Could you check a few things on this model? Use its own coordinates, in mm. A direction names the side the tool comes from. Give positions to 0.01 mm unless a question says otherwise; leave off trailing zeros. Order: outer loops, then holes, each group sorted by start corner. A loop starts at its lowest first (then second) coordinate and runs counter-clockwise, first axis right, second up. Notation, with made-up numbers: (22.5, -32) -> (59.5, -32) arc R17 cw to (59.5, -21) -> close; hole circle Ø6 at (52, 22). An arc over 180 degrees is marked (long way). Write each question's results on one line, items separated by ' | '.
```python
from build123d import *

# Parameters (mm, degrees)
F3_DEPTH      = 40.001
F3_DEPTH_BACK = 40.001
F4_R          = 20
F5_DEPTH      = 40.001
F5_DEPTH_BACK = 40.001


with BuildPart() as f1:
    # F0 (on Front) → F1 (revolve)
    with BuildSketch(Plane.XZ):
        with BuildLine():
            ThreePointArc((0, 40), (-40, 0), (0, -40))
            Line((0, -40), (0, 40))
        make_face()
    revolve(axis=Axis((0, 0, 0), (0, 0, 1)))

    # F2 (on Front) → F3 (cut, two sides)
    with BuildSketch(Plane.XZ) as f3_sk:
        Polygon((12.5, -25.9565174572), (28.0872450465, -6.4107303955), (22.5242216976, 17.9624674091), (0, 28.809560887), (-22.5242216976, 17.9624674091), (-28.0872450465, -6.4107303955), (-12.5, -25.9565174572), align=None)
    extrude(amount=-F3_DEPTH, mode=Mode.SUBTRACT)
    extrude(f3_sk.sketch, amount=F3_DEPTH_BACK, mode=Mode.SUBTRACT)

    # F4 (on Right) → F5 (cut, two sides)
    with BuildSketch(Plane.YZ) as f5_sk:
        Circle(F4_R)
    extrude(amount=-F5_DEPTH, mode=Mode.SUBTRACT)
    extrude(f5_sk.sketch, amount=F5_DEPTH_BACK, mode=Mode.SUBTRACT)


solid = f1.part
```
Q1. I need wall thicknesses on line 1 along Z through (x, y) = (-6, -11); line 2 along Z through (x, y) = (-25, 2); line 3 along X through (y, z) = (-26.5, 9). Which ranges of each line are inside material? Lowest first, please.
Here are the results:
line 1: z = -37.99 to -25.96, 25.92 to 37.99 | line 2: z = -31.16 to -19.9, 19.9 to 31.16 | line 3: x = -28.58 to -24.57, 24.57 to 28.58
Q2. Suppose I cut it at A-A on z = -11. Please give me the cut outline in (x, y).
Here are the results:
outline: (-34.64, -16.7) arc R38.46 ccw to (-24.43, -29.7) -> (-24.43, -16.7) -> close; (-34.64, 16.7) -> (-24.43, 16.7) -> (-24.43, 29.7) arc R38.46 ccw to start; (24.43, -29.7) arc R38.46 ccw to (34.64, -16.7) -> (24.43, -16.7) -> close; (24.43, 16.7) -> (34.64, 16.7) arc R38.46 ccw to (24.43, 29.7) -> close
Q3. Suppose I cut it at D-D on y = 4.5. Please give me the cut outline in (x, z), and give its area (3 significant figures).
Here are the results:
outline: (-34.64, -19.49) arc R39.75 ccw to (34.64, -19.49) -> (17.66, -19.49) -> (12.5, -25.96) -> (-12.5, -25.96) -> (-17.66, -19.49) -> close; (-34.64, 19.49) -> (-19.36, 19.49) -> (0, 28.81) -> (19.36, 19.49) -> (34.64, 19.49) arc R39.75 ccw to start | area: 1,620 mm²
Q4. For faces 3 (the flat face through (-11.104, 0.426, 23.462)), 4 (the cylindrical face through (-27.756, -4.336, -19.524)), which set-ups out of +Z, -Z, +X, -X, +Y, -Y let a thin tool reach every point of the face, with its end or its side?
Here are the results:
face 3: +Y, -Y | face 4: +X, -X
Q5. Suppose I cut it at B-B on x = 19.5. Please give me the cut outline in (y, z), and give its area (3 significant figures).
Here are the results:
outline: (-30.41, -17.18) arc R34.92 ccw to (30.41, -17.18) -> (10.24, -17.18) arc R20 cw to (-10.24, -17.18) -> close; (-29.03, 19.42) -> (-4.79, 19.42) arc R20 cw to (4.79, 19.42) -> (29.03, 19.42) arc R34.92 ccw to start | area: 1,360 mm²
Q6. I'm going to push flat-ended pins straight in: pin 1 Ø4 at (x, z) = (3, 32) entering from +Y; pin 2 Ø3 at (x, y) = (-12, -20.5) entering from +Z; pin 3 Ø10 at (x, y) = (-11.5, -0.5) entering from +Z. Where does each tip first touch, or does it pass through?
Here are the results:
pin 1: stops at y = 26.3 | pin 2: stops at z = 33.24 | pin 3: stops at z = 39.47
Q7. Thinking about a two-plate mould opening in Y: for faces 1 (the flat face through (-16.94, 0.43, -20.39)), 2 (the cylindrical face through (27.756, -4.336, -19.524)), which applies, +Y half, -Y half, draft (parallel to the pull), parting line (faces both ways), or undercut?
Here are the results:
face 1: draft | face 2: undercut
Q8. Suppose I cut it at C-C on y = -16. Please give me the cut outline in (x, z), and give its area (3 significant figures).
Here are the results:
outline: (-34.64, -12) arc R36.66 ccw to (34.64, -12) -> (23.63, -12) -> (12.5, -25.96) -> (-12.5, -25.96) -> (-23.63, -12) -> close; (-34.64, 12) -> (-23.89, 12) -> (-22.52, 17.96) -> (0, 28.81) -> (22.52, 17.96) -> (23.89, 12) -> (34.64, 12) arc R36.66 ccw to start | area: 1,470 mm²
